```python
from build123d import *

# Parameters (mm, degrees)
SKETCH1_W           = 200
SKETCH1_H           = 200
SKETCH1_R           = 2
BOSS_EXTRUDE1_DEPTH = 4
FILLET1_R           = 10
SKETCH2_W           = 332.366301243
SKETCH2_H           = 358.749780036
CUT_EXTRUDE1_DEPTH  = 10


with BuildPart() as part:
    # Sketch1 → Boss-Extrude1 (new body)
    with BuildSketch(Plane(origin=(0, 0, 0), x_dir=(1, 0, 0), z_dir=(0, 1, 0))):
        Rectangle(SKETCH1_W, SKETCH1_H)
        Circle(SKETCH1_R, mode=Mode.SUBTRACT)
    extrude(amount=BOSS_EXTRUDE1_DEPTH)

    # Fillet1
    fillet1_edges = [part.edges().sort_by_distance(p)[0] for p in [
        (-100, 2, -100),
        (100, 2, -100),
        (100, 2, 100),
        (-100, 2, 100),
    ]]
    fillet(fillet1_edges, radius=FILLET1_R)

    # Sketch2 → Cut-Extrude1 (cut)
    with BuildSketch(Plane(origin=(0, 4, 0), x_dir=(1, 0, 0), z_dir=(0, 1, 0))):
        with Locations((1.781411531, 2.248264207)):
            Rectangle(SKETCH2_W, SKETCH2_H)
        with BuildLine():
            Line((-62.5, 91.5), (62.5, 91.5))
            ThreePointArc((62.5, 91.5), (69.571067812, 88.571067812), (72.5, 81.5))
            Line((72.5, 81.5), (72.5, -81.5))
            ThreePointArc((72.5, -81.5), (69.571067812, -88.571067812), (62.5, -91.5))
            Line((62.5, -91.5), (-62.5, -91.5))
            ThreePointArc((-62.5, -91.5), (-69.571067812, -88.571067812), (-72.5, -81.5))
            Line((-72.5, -81.5), (-72.5, 81.5))
            ThreePointArc((-72.5, 81.5), (-69.571067812, 88.571067812), (-62.5, 91.5))
        make_face(mode=Mode.SUBTRACT)
    extrude(amount=-CUT_EXTRUDE1_DEPTH, mode=Mode.SUBTRACT)


solid = part.part
```
Can you work these out from the model? Positions are in its coordinate system, mm. Coordinates: 2 decimals unless noted, no trailing zeros. Write each loop counter-clockwise with the first axis right and the second up, starting at its lowest first coordinate (ties: lowest second). Pieces come first, ordered by that corner, then holes. Notation, with made-up numbers: M 50.5,-17.5 L 63.5,-17.5 A30 ccw 63.5,5.5 Z; hole C -6.5,48 d5. An arc over 180 degrees is marked long. Answer as CSV lines item,"result".
Item 1: Imagine slicing it at B-B on z = 0. List the corners of the cut face in (x, y) for me.
Geometry results:
outline,"M -72.5,0 L -2,0 L -2,4 L -72.5,4 Z; M 2,0 L 72.5,0 L 72.5,4 L 2,4 Z"
Item 2: Imagine slicing it at A-A on x = 0. List the corners of the cut face in (y, z) for me, plus the area to 3 significant figures.
Geometry results:
outline,"M 0,-91.5 L 4,-91.5 L 4,-2 L 0,-2 Z; M 0,2 L 4,2 L 4,91.5 L 0,91.5 Z"
area,"716 mm2"
Item 3: Please list where these lines run through material, in increasing order: line 1 along X through (y, z) = (1.85, 0); line 2 along Z through (x, y) = (0, 1.2); line 3 along Z through (x, y) = (0.5, 1.8).
Geometry results:
line 1,"x = -72.5 to -2, 2 to 72.5"
line 2,"z = -91.5 to -2, 2 to 91.5"
line 3,"z = -91.5 to -1.94, 1.94 to 91.5"
Item 4: We'd pull the mould along Z, two halves only. Please class faces 1 (the flat face through (15, 4, -1)), 2 (the cylindrical face through (0, 2, 2)), 3 (the cylindrical face through (-69.49, 2.03, 88.65)): +Z half, -Z half, draft (parallel to the pull), parting line (faces both ways), or undercut.
Geometry results:
face 1,"draft"
face 2,"undercut"
face 3,"+Z half"
